```python
from build123d import *

# Parameters (mm, degrees)
F0_W     = 31.1658
F0_H     = 76.073
F1_DEPTH = 2.0955
F2_W     = 12.192
F2_H     = 2.0955
F2_W_2   = 16.637
F3_DEPTH = 1.9558
F4_R     = 5.2705
F5_DEPTH = 12.192
F7_DEPTH = 16.637
F9_DEPTH = 12.192


with BuildPart() as f1:
    # F0 (on Top) → F1 (new body)
    with BuildSketch(Plane.XY):
        Rectangle(F0_W, F0_H)
    extrude(amount=F1_DEPTH)

    # F2 (on face) → F3 (join)
    with BuildSketch(Plane.YZ.offset(15.5829)):
        with Locations((-31.9405, 1.04775)):
            Rectangle(F2_W, F2_H)
        with Locations((0, 1.04775)):
            Rectangle(F2_W_2, F2_H)
        with Locations((31.9405, 1.04775)):
            Rectangle(F2_W, F2_H)
    extrude(amount=F3_DEPTH)

    # F4 (on face) → F5 (join, through all)
    with BuildSketch(Plane.XZ.offset(38.0365)):
        with Locations((22.1742, -0.9652)):
            Circle(F4_R)
    extrude(amount=-F5_DEPTH)

    # F6 (on face) → F7 (join, through all)
    with BuildSketch(Plane.XZ.offset(8.3185)):
        with BuildLine():
            Line((17.5387, 0), (16.992833, 0))
            ThreePointArc((16.992833, 0), (27.024756, -3.026821), (17.883479, 2.0955))
            Line((17.883479, 2.0955), (17.5387, 2.0955))
            Line((17.5387, 2.0955), (17.5387, 0))
        make_face()
    extrude(amount=-F7_DEPTH)

    # F8 (on face) → F9 (join, through all)
    with BuildSketch(Plane.XZ.offset(-25.8445)):
        with BuildLine():
            Line((17.5387, 0), (16.992833, 0))
            ThreePointArc((16.992833, 0), (27.024756, -3.026821), (17.883479, 2.0955))
            Line((17.883479, 2.0955), (17.5387, 2.0955))
            Line((17.5387, 2.0955), (17.5387, 0))
        make_face()
    extrude(amount=-F9_DEPTH)


solid = f1.part
```
Here's how the part is built. I have some questions about the finished solid (model axes, mm). A direction names the side the tool comes from. Coordinates: 2 decimals unless noted, no trailing zeros. Write each loop counter-clockwise with the first axis right and the second up, starting at its lowest first coordinate (ties: lowest second). Pieces come first, ordered by that corner, then holes. Notation, with made-up numbers: M 10.25,-4 L 69.25,-4 A18 ccw 69.25,22 Z; hole C 28.5,75 d2. An arc over 180 degrees is marked long. Answer as CSV lines item,"result". Start each with the question number.
Q1. For faces 1 (the flat face through (21, -8.318, -1)), 2 (the flat face through (-15.583, -1, 1)), 3 (the flat face through (1, -1, 2.096)), which set-ups out of +Z, -Z, +X, -X, +Y, -Y let a thin tool reach every point of the face, with its end or its side?
Q2. I need wall thicknesses on probe 1 along Y at (x, z) = (19, 0.25); probe 2 along Z at (x, y) = (0, -5); probe 3 along X at (y, z) = (19.5, 1.5). Which ranges of each line are inside material? Lowest first, please. Write a range as [from, to].
Q3. Suppose I cut it at D-D, the plane x = 7. List the corners of the cut face in (y, z) for me.
Q4. Will these pins go through, and if not, where does the flat tip stop? pin 1 Ø2 at (x, y) = (-4, 22) entering from +Z; pin 2 Ø1.5 at (y, z) = (-6.5, -5) entering from +X; pin 3 Ø0.6 at (y, z) = (-21, 1.5) entering from +X.
Q5. Suppose I cut it at A-A, the plane z = -3. List the corners of the cut face in (x, y) for me.
Q6. Suppose I cut it at B-B, the plane x = 19. List the corners of the cut face in (y, z) for me.
Q7. Suppose I cut it at C-C, the plane y = -31. List the corners of the cut face in (x, z) for me.
Entries:
1,face 1,"+Z, -Z, +X"
1,face 2,"+Z, -Z, -X, +Y, -Y"
1,face 3,"+Z, -X, +Y, -Y"
2,probe 1,"y = [-38.04, -25.84], [-8.32, 8.32], [25.84, 38.04]"
2,probe 2,"z = [0, 2.1]"
2,probe 3,"x = [-15.58, 15.58]"
3,outline,"M -38.04,0 L 38.04,0 L 38.04,2.1 L -38.04,2.1 Z"
4,pin 1,"stops at z = 2.1"
4,pin 2,"stops at x = 26.3"
4,pin 3,"stops at x = 15.58"
5,outline,"M 17.31,-38.04 L 27.04,-38.04 L 27.04,-25.84 L 17.31,-25.84 Z; M 17.31,-8.32 L 27.04,-8.32 L 27.04,8.32 L 17.31,8.32 Z; M 17.31,25.84 L 27.04,25.84 L 27.04,38.04 L 17.31,38.04 Z"
6,outline,"M -38.04,-5.17 L -25.84,-5.17 L -25.84,3.24 L -38.04,3.24 Z; M -8.32,-5.17 L 8.32,-5.17 L 8.32,3.24 L -8.32,3.24 Z; M 25.84,-5.17 L 38.04,-5.17 L 38.04,3.24 L 25.84,3.24 Z"
7,outline,"M -15.58,0 L 16.99,0 A5.27 ccw long 17.54,1.54 L 17.54,2.1 L -15.58,2.1 Z"
